Check sheet for the drawn part. Datum: minimum x, y, z corner. Units: mm. Round coordinates to 2 decimals unless told otherwise and drop trailing zeros. Write each loop counter-clockwise with the first axis right and the second up, starting at its lowest first coordinate (ties: lowest second). Pieces come first, ordered by that corner, then holes. Notation, with made-up numbers: M 4,84.25 L 37,84.25 A23 ccw 37,116.25 Z; hole C -14,54 d1. An arc over 180 degrees is marked long. Put each result on its own line as item: value.
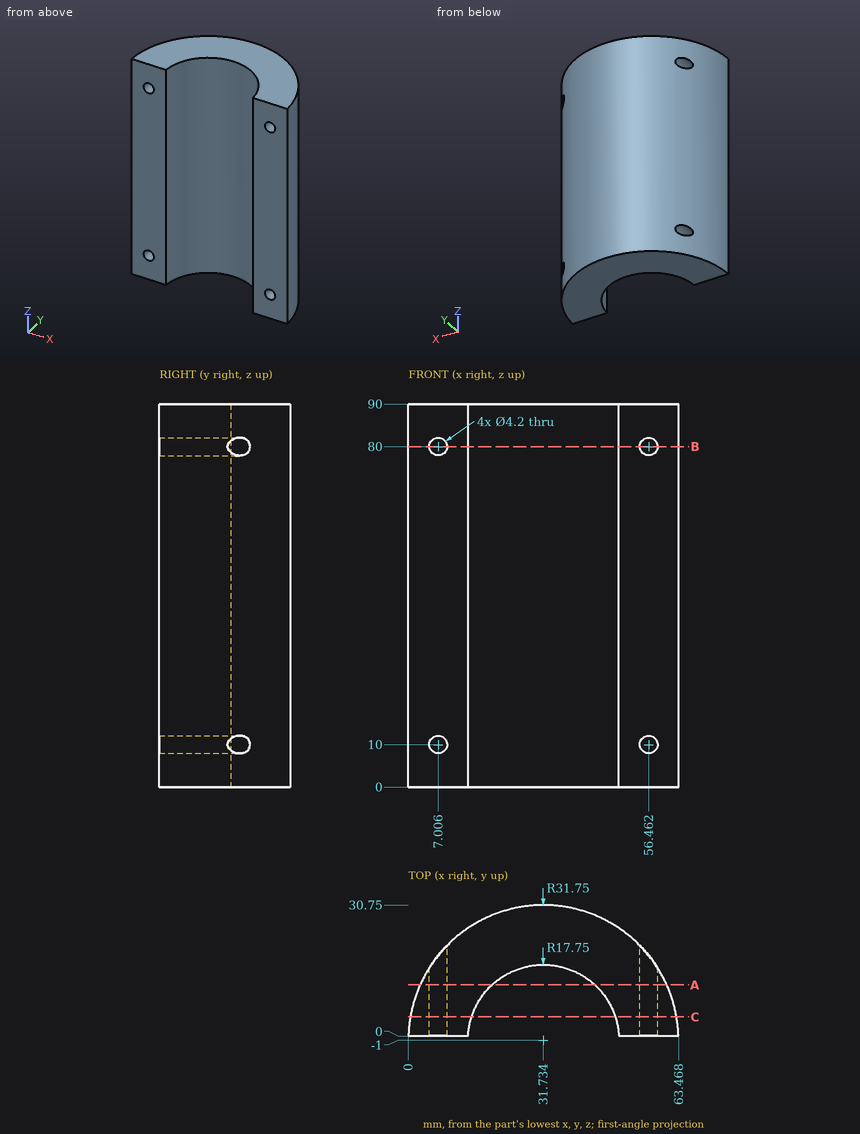
1. Cross-section at A-A (y = 12). Enter the section's corners in (x, z), then the cut area to 3 significant figures.
Computed values:
outline: M 2.77,0 L 19.65,0 L 19.65,90 L 2.77,90 Z; M 43.82,0 L 60.7,0 L 60.7,90 L 43.82,90 Z; hole C 7.01,10 d4.2; hole C 7.01,80 d4.2; hole C 56.46,10 d4.2; hole C 56.46,80 d4.2
area: 2,980 mm2
2. Cross-section at B-B (z = 80). Count the separate pieces of the cut face and the enclosed holes in it.
Computed values:
separate pieces: 3
enclosed holes: 0
3. Scan lines: probe 1 along Z at (x, y) = (6.5, 2.5); probe 2 along X at (y, z) = (8, 10) (1 decimal); probe 3 along X at (y, z) = (6, 80) (1 decimal). Record each from-to range of solid material in increasing order.
Computed values:
probe 1: z = 0 to 7.96, 12.04 to 77.96, 82.04 to 90
probe 2: x = 1.3 to 4.9, 9.1 to 16.4, 47 to 54.4, 58.6 to 62.2
probe 3: x = 0.8 to 4.9, 9.1 to 15.4, 48 to 54.4, 58.6 to 62.7
4. Cross-section at C-C (y = 4.5). Enter the section's corners in (x, z) (1 decimal).
Computed values:
outline: M 0.5,0 L 14.9,0 L 14.9,90 L 0.5,90 Z; M 48.6,0 L 63,0 L 63,90 L 48.6,90 Z; hole C 7,10 d4.2; hole C 7,80 d4.2; hole C 56.5,10 d4.2; hole C 56.5,80 d4.2
5. Depth check by flat-ended pin: pin 1 Ø10 at (y, z) = (20.5, 81) entering from +X; pin 2 Ø6 at (y, z) = (27, 70) entering from +X (1 decimal); pin 3 Ø3 at (x, z) = (42.5, 13.5) entering from +Y. Enter the tip coordinate at first touch or a pass-through.
Computed values:
pin 1: stops at x = 58.86
pin 2: stops at x = 51.3
pin 3: stops at y = 29.37
